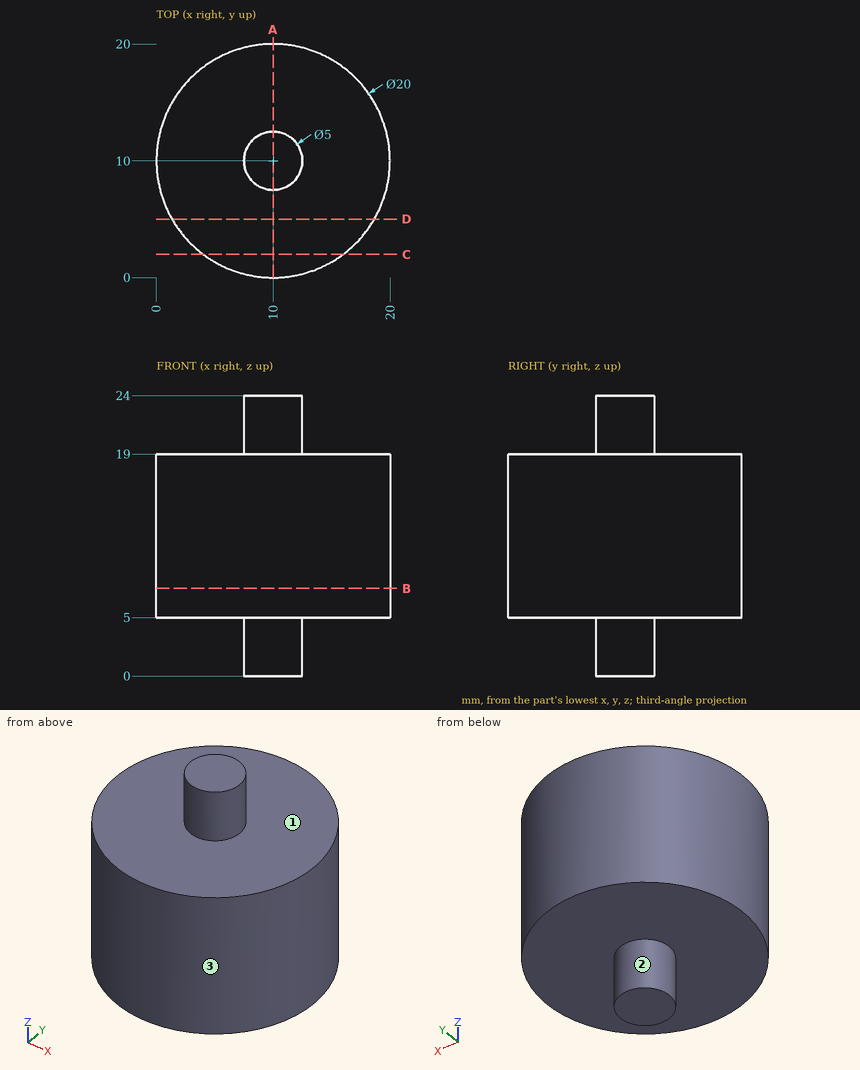
Study the drawing (mm; zero at the part's minimum x, y, z) and answer. A direction names the side the tool comes from. Give positions to 0.01 mm unless a question says otherwise; leave off trailing zeros. Write each loop counter-clockwise with the first axis right and the second up, starting at its lowest first coordinate (ties: lowest second). Pieces come first, ordered by that corner, then holes. Notation, with made-up numbers: (53.25, -36.5) - (88.25, -36.5) arc R10 cw to (88.25, -25.5) - close; hole circle Ø2 at (18.25, 88.5). An arc over 180 degrees is marked (long way). Write item = value, one per line. Start each with the question number.
Item 1: Find section B-B (z = 7.5). Give the vertices of the cut face in (x, y), then the cut area to 3 significant figures.
Item 2: Each of these flat-tipped pins is pushed along its axis until it touches: P1, Ø8, axis at x = 3.5, y = 9, coming from the -Z side; P2, Ø2, axis at y = 12.5, z = 12.5, coming from the -X side; P3, Ø1, axis at y = 11, z = 15.5, coming from the -X side. Where does it stop, or does it pass through?
Item 3: Find the intervals of material crossed by probe 1 along X at (y, z) = (10, 2.25); probe 2 along Z at (x, y) = (16.5, 15.5); probe 3 along X at (y, z) = (9.75, 15.25), in increasing order. Write a range as [from, to].
Item 4: Find section A-A (x = 10). Give the vertices of the cut face in (y, z), then the cut area to 3 significant figures.
Item 5: Find section C-C (y = 2). Give the vertices of the cut face in (x, z).
Item 6: Find section D-D (y = 5). Give the vertices of the cut face in (x, z), then the cut area to 3 significant figures.
Item 7: A tool of negligible diameter and unlimited length cuts with its end or side. For the marked faces 1, 2 and 3, from which of +Z, -Z, +X, -X, +Y, -Y can it reach the whole face along a straight path? Write none if from no direction.
Response:
q1.outline = circle Ø20 at (10, 10)
q1.area = 314 mm²
q2.P1 = 5
q2.P2 = 0.11
q2.P3 = 0.01
q3.probe_1 = [7.5, 12.5]
q3.probe_2 = [5, 19]
q3.probe_3 = [0, 20]
q4.outline = (0, 5) - (7.5, 5) - (7.5, 0) - (12.5, 0) - (12.5, 5) - (20, 5) - (20, 19) - (12.5, 19) - (12.5, 24) - (7.5, 24) - (7.5, 19) - (0, 19) - close
q4.area = 330 mm²
q5.outline = (4, 5) - (16, 5) - (16, 19) - (4, 19) - close
q6.outline = (1.34, 5) - (18.66, 5) - (18.66, 19) - (1.34, 19) - close
q6.area = 242 mm²
q7.face_1 = +Z
q7.face_2 = -Z
q7.face_3 = +Z, -Z
